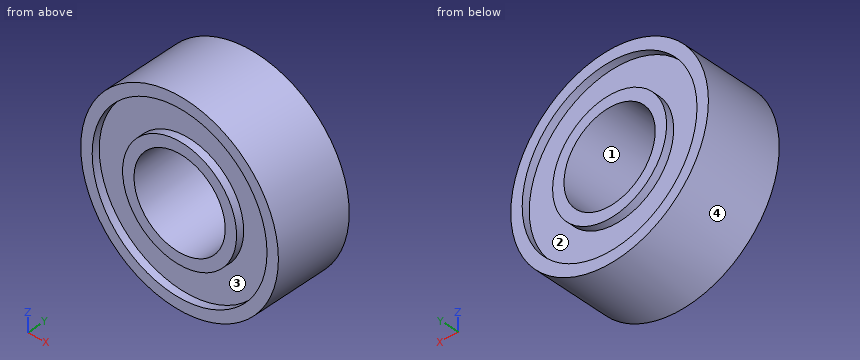
Autodesk Inventor part; units mm, degrees
ref_plane "YZ Plane" through (0, 0, 0) normal (1, 0, 0) x (0, 1, 0)
ref_plane "XZ Plane" through (0, 0, 0) normal (0, 1, 0) x (-1, 0, 0)
ref_plane "XY Plane" through (0, 0, 0) normal (0, 0, 1) x (1, 0, 0)
sketch "草图1" plane through (0, 0, 0) normal (0, 1, 0) x (-1, 0, 0)
  circle A0 centre (0, 0) radius 6.5
  circle A1 centre (0, 0) radius 3
  dimension "d0" = 13
  dimension "d1" = 6
extrude "拉伸1" add sketch "草图1" along normal blind 5
sketch "草图2" plane through (0, 5, 0) normal (0, 1, 0) x (1, 0, 0)
  circle A0 centre (0, 0) radius 3
  circle A1 centre (0, 0) radius 6.5
  circle A2 centre (0, 0) radius 3.75
  circle A3 centre (0, 0) radius 5.75
  dimension "d4" = 11.5
  dimension "d5" = 7.5
extrude "拉伸2" cut sketch "草图2" against normal blind 0.5 contours A3
sketch "草图3" plane through (0, 0, 0) normal (0, -1, 0) x (1, 0, 0)
  circle A0 centre (0, 0) radius 3.75
  circle A1 centre (0, 0) radius 5.75
extrude "拉伸3" cut sketch "草图3" against normal blind 0.5
properties part number "bearing_6_13_5"
Here's how the part is built. I have some questions about the finished solid (model axes, mm). Face numbers are marked on the shaded views. A direction names the side the tool comes from. Give positions to 0.01 mm unless a question says otherwise; leave off trailing zeros. Write each loop counter-clockwise with the first axis right and the second up, starting at its lowest first coordinate (ties: lowest second). Pieces come first, ordered by that corner, then holes. Notation, with made-up numbers: (61, 56.5) -> (65, 56.5) arc R24 cw to (65, 67.5) -> close; hole circle Ø9 at (66.25, 49). An arc over 180 degrees is marked (long way). Write each question's results on one line, items separated by ' | '.
Item 1: On a 3-axis mill with a long thin cutter (end or side, diameter ignored), from which of +Z, -Z, +X, -X, +Y, -Y can I reach the whole of each face in a straight line? I mean the marked faces 1 and 2. Say none if no direction works.
Output:
face 1: +Y, -Y | face 2: +Y
Item 2: For pin 1 Ø1 at (x, y) = (1.5, 3.5) entering from +Z; pin 2 Ø1.5 at (x, z) = (0, 2) entering from +Y; pin 3 Ø2 at (x, y) = (-4, 1) entering from -Z; pin 4 Ø1 at (y, z) = (1, -3.5) entering from -X, each with a flat end and sliding along its axis, tell me the tip position at first contact or that it passes through.
Output:
pin 1: stops at z = 6.42 | pin 2: passes through | pin 3: stops at z = -5.77 | pin 4: stops at x = -5.77
Item 3: Suppose I cut it at B-B on z = 0. Write out the boundary of the cut face in (x, y), plus the area to 3 significant figures.
Output:
outline: (-6.5, 0) -> (-5.75, 0) -> (-5.75, 0.5) -> (-3.75, 0.5) -> (-3.75, 0) -> (-3, 0) -> (-3, 5) -> (-3.75, 5) -> (-3.75, 4.5) -> (-5.75, 4.5) -> (-5.75, 5) -> (-6.5, 5) -> close; (3, 0) -> (3.75, 0) -> (3.75, 0.5) -> (5.75, 0.5) -> (5.75, 0) -> (6.5, 0) -> (6.5, 5) -> (5.75, 5) -> (5.75, 4.5) -> (3.75, 4.5) -> (3.75, 5) -> (3, 5) -> close | area: 31.0 mm^2
Item 4: Suppose I cut it at C-C on y = 2.65. Write out the boundary of the cut face in (x, z), plus the area to 3 significant figures.
Output:
outline: circle Ø13 at (0, 0); hole circle Ø6 at (0, 0) | area: 104 mm^2
Item 5: If I drill on L1, parallel to Z at x = 0, y = 0.2; L2, parallel to Z at x = 0, y = 3.7; L3, parallel to X at y = 0.25, z = -1.25, over which ranges is the centre line in solid material (lowest first)?
Output:
L1: z = -6.5 to -5.75, -3.75 to -3, 3 to 3.75, 5.75 to 6.5 | L2: z = -6.5 to -3, 3 to 6.5 | L3: x = -6.38 to -5.61, -3.54 to -2.73, 2.73 to 3.54, 5.61 to 6.38
Item 6: Suppose I cut it at D-D on x = 5. Write out the boundary of the cut face in (y, z).
Output:
outline: (0, -4.15) -> (5, -4.15) -> (5, -2.84) -> (4.5, -2.84) -> (4.5, 2.84) -> (5, 2.84) -> (5, 4.15) -> (0, 4.15) -> (0, 2.84) -> (0.5, 2.84) -> (0.5, -2.84) -> (0, -2.84) -> close
Item 7: Suppose I cut it at A-A on x = 0. Write out the boundary of the cut face in (y, z).
Output:
outline: (0, -6.5) -> (5, -6.5) -> (5, -5.75) -> (4.5, -5.75) -> (4.5, -3.75) -> (5, -3.75) -> (5, -3) -> (0, -3) -> (0, -3.75) -> (0.5, -3.75) -> (0.5, -5.75) -> (0, -5.75) -> close; (0, 3) -> (5, 3) -> (5, 3.75) -> (4.5, 3.75) -> (4.5, 5.75) -> (5, 5.75) -> (5, 6.5) -> (0, 6.5) -> (0, 5.75) -> (0.5, 5.75) -> (0.5, 3.75) -> (0, 3.75) -> close
Item 8: We'd pull the mould along Z, two halves only. Please class the marked faces 3 and 4: pulls with the +Z half, pulls with the -Z half, needs draft (parallel to the pull), parting line crosses it, or undercut.
Output:
face 3: undercut | face 4: parting line crosses it
